Geometry check sheet. Reference: the model listing, model coordinates, mm. Round coordinates to 2 decimals unless told otherwise and drop trailing zeros. Order: outer loops, then holes, each group sorted by start corner. A loop starts at its lowest first (then second) coordinate and runs counter-clockwise, first axis right, second up. Notation, with made-up numbers: M -7.75,-36 L 2.25,-36 A14 ccw 2.25,-21 Z; hole C 37,17 d4. An arc over 180 degrees is marked long. Return JSON: item names as keys, results as strings. Group by question number.
```python
from build123d import *

# Parameters (mm, degrees)
SKETCH1_W           = 117
SKETCH1_H           = 27
SKETCH1_R           = 3.5
BOSS_EXTRUDE1_DEPTH = 2.5
FILLET1_R           = 1


with BuildPart() as part:
    # Sketch1 → Boss-Extrude1 (new body, symmetric)
    with BuildSketch(Plane.XY):
        with Locations((58.5, 13.5)):
            Rectangle(SKETCH1_W, SKETCH1_H)
        with Locations((13.5, 13.5)):
            Circle(SKETCH1_R, mode=Mode.SUBTRACT)
        with Locations((43.5, 13.5)):
            Circle(SKETCH1_R, mode=Mode.SUBTRACT)
        with Locations((73.5, 13.5)):
            Circle(SKETCH1_R, mode=Mode.SUBTRACT)
        with Locations((103.5, 13.5)):
            Circle(SKETCH1_R, mode=Mode.SUBTRACT)
    extrude(amount=BOSS_EXTRUDE1_DEPTH, both=True)

    # Fillet1
    fillet1_edges = [part.edges().sort_by_distance(p)[0] for p in [
        (58.5, 27, 2.5),
        (0, 13.5, 2.5),
        (58.5, 0, 2.5),
        (117, 13.5, 2.5),
        (0, 0, 0),
        (0, 27, 0),
        (117, 27, 0),
        (117, 0, 0),
    ]]
    fillet(fillet1_edges, radius=FILLET1_R)


solid = part.part
```
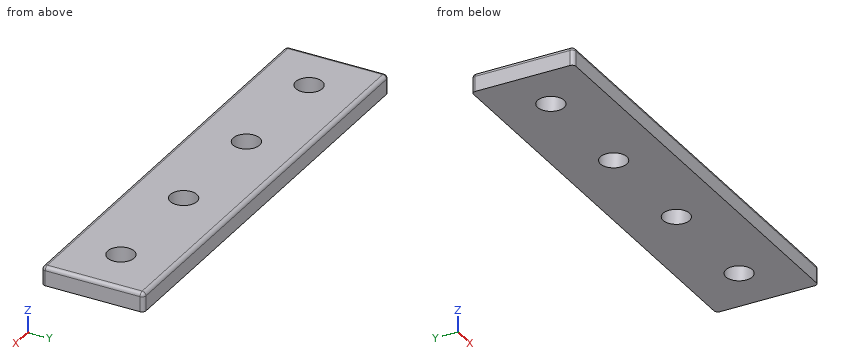
Q1. Material ranges on line 1 along Y through (x, z) = (103.5, 1.45); line 2 along X through (y, z) = (12.5, 1.7); line 3 along Y through (x, z) = (106, 1.7), recorded low to high.
Q2. Section check B-B on z = -1.45. Record the cut outline in (x, y), plus the area to 3 significant figures.
Q3. Section check C-C on x = 73.5. Record the cut outline in (y, z).
Q4. Section check A-A on y = 13.5. Record the cut outline in (x, z), plus the area to 3 significant figures.
Q5. Depth check by flat-ended pin: pin 1 Ø4 at (x, y) = (103.5, 13.5) entering from -Z. Enter the tip coordinate at first touch or a pass-through.
Q6. Section check D-D on x = 41.5. Record the cut outline in (y, z), plus the area to 3 significant figures.
Geometry check:
{
 "1": {"line 1": "y = 0 to 10, 17 to 27", "line 2": "x = 0.02 to 10.15, 16.85 to 40.15, 46.85 to 70.15, 76.85 to 100.15, 106.85 to 116.98", "line 3": "y = 0.02 to 11.05, 15.95 to 26.98"},
 "2": {"outline": "M 0,1 A1 ccw 1,0 L 116,0 A1 ccw 117,1 L 117,26 A1 ccw 116,27 L 1,27 A1 ccw 0,26 Z; hole C 13.5,13.5 d7; hole C 43.5,13.5 d7; hole C 73.5,13.5 d7; hole C 103.5,13.5 d7", "area": "3,000 mm^2"},
 "3": {"outline": "M 0,-2.5 L 10,-2.5 L 10,2.5 L 1,2.5 A1 ccw 0,1.5 Z; M 17,-2.5 L 27,-2.5 L 27,1.5 A1 ccw 26,2.5 L 17,2.5 Z"},
 "4": {"outline": "M 0,-2.5 L 10,-2.5 L 10,2.5 L 1,2.5 A1 ccw 0,1.5 Z; M 17,-2.5 L 40,-2.5 L 40,2.5 L 17,2.5 Z; M 47,-2.5 L 70,-2.5 L 70,2.5 L 47,2.5 Z; M 77,-2.5 L 100,-2.5 L 100,2.5 L 77,2.5 Z; M 107,-2.5 L 117,-2.5 L 117,1.5 A1 ccw 116,2.5 L 107,2.5 Z", "area": "445 mm^2"},
 "5": {"pin 1": "passes through"},
 "6": {"outline": "M 0,-2.5 L 10.63,-2.5 L 10.63,2.5 L 1,2.5 A1 ccw 0,1.5 Z; M 16.37,-2.5 L 27,-2.5 L 27,1.5 A1 ccw 26,2.5 L 16.37,2.5 Z", "area": "106 mm^2"}
}
